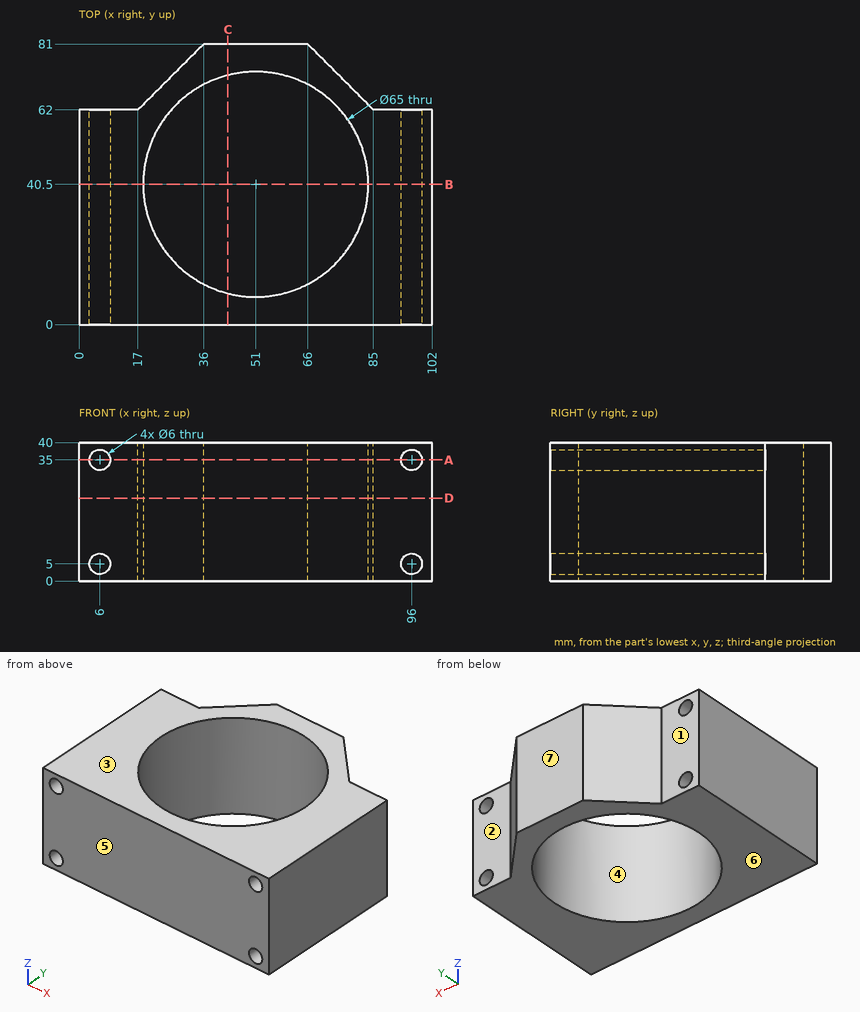
Design review of the part shown in the three views and the two pictorial views. Dimensions are in mm from the part's minimum x, y and z. A direction names the side the tool comes from. Coordinates: 2 decimals unless noted, no trailing zeros. Write each loop counter-clockwise with the first axis right and the second up, starting at its lowest first coordinate (ties: lowest second). Pieces come first, ordered by that corner, then holes.
1) We need section D-D on z = 24. State the section outline as (x, y) points, then the cut area to 3 significant figures.
2) Machinability: for the marked faces 1, 2 and 3, which of the approach directions +Z, -Z, +X, -X, +Y, -Y give a long, thin tool a straight path to every point of the face, cutting with its end or side? Answer none if there is none.
3) The part is to be moulded in two halves that separate along Y. For the marked faces 4, 5, 6 and 7, say which applies: pulls with the +Y half, pulls with the -Y half, needs draft (parallel to the pull), parting line crosses it, or undercut.
4) We need section B-B on y = 40.5. State the section outline as (x, z) points, then the cut area to 3 significant figures.
5) We need section A-A on z = 35. State the section outline as (x, y) points, then the cut area to 3 significant figures.
6) We need section C-C on x = 43. State the section outline as (y, z) points.
7) To check wall thickness, follow probe 1 along Z at (x, y) = (6, 34); probe 2 along X at (y, z) = (30, 5); probe 3 along X at (y, z) = (20, 35). State the ranges of each line that lie inside material, in increasing order.
8) Clearance check with a flat-ended pin moving along its axis: pin 1 Ø9.5 at (x, z) = (6, 5) entering from +Y. State where the tip first meets the part, or that it passes through.
Answer list:
1. outline: (0, 0) - (102, 0) - (102, 62) - (85, 62) - (66, 81) - (36, 81) - (17, 62) - (0, 62) - close; hole circle Ø65 at (51, 40.5)
1. area: 3,940 mm2
2. face 1: +Z, -Z, -X, +Y
2. face 2: +Z, -Z, +X, +Y
2. face 3: +Z, +X, -X, +Y, -Y
3. face 4: undercut
3. face 5: pulls with the -Y half
3. face 6: needs draft
3. face 7: pulls with the +Y half
4. outline: (0, 0) - (18.5, 0) - (18.5, 40) - (0, 40) - close; (83.5, 0) - (102, 0) - (102, 40) - (83.5, 40) - close; hole circle Ø6 at (6, 5); hole circle Ø6 at (6, 35); hole circle Ø6 at (96, 5); hole circle Ø6 at (96, 35)
4. area: 1,370 mm2
5. outline: (0, 0) - (3, 0) - (3, 62) - (0, 62) - close; (9, 0) - (93, 0) - (93, 62) - (85, 62) - (66, 81) - (36, 81) - (17, 62) - (9, 62) - close; (99, 0) - (102, 0) - (102, 62) - (99, 62) - close; hole circle Ø65 at (51, 40.5)
5. area: 3,190 mm2
6. outline: (0, 0) - (9, 0) - (9, 40) - (0, 40) - close; (72, 0) - (81, 0) - (81, 40) - (72, 40) - close
7. probe 1: z = 0 to 2, 8 to 32, 38 to 40
7. probe 2: x = 0 to 3, 9 to 20.24, 81.76 to 93, 99 to 102
7. probe 3: x = 0 to 3, 9 to 25.78, 76.22 to 93, 99 to 102
8. pin 1: stops at y = 62
